```python
from build123d import *

# Parameters (mm, degrees)
ESQUISSE1_R      = 72.5
ESQUISSE1_R_2    = 5
ESQUISSE1_R_3    = 2
EXTRUSION1_DEPTH = 30


with BuildPart() as part:
    # Esquisse1 → Extrusion1 (new body)
    with BuildSketch(Plane.XY):
        Circle(ESQUISSE1_R)
        with Locations((0, -65)):
            Circle(ESQUISSE1_R_2, mode=Mode.SUBTRACT)
        with Locations((65, 0)):
            Circle(ESQUISSE1_R_2, mode=Mode.SUBTRACT)
        with Locations((0, 65)):
            Circle(ESQUISSE1_R_2, mode=Mode.SUBTRACT)
        with Locations((32.5, 56.291651246)):
            Circle(ESQUISSE1_R_3, mode=Mode.SUBTRACT)
        with Locations((-32.5, -56.291651246)):
            Circle(ESQUISSE1_R_3, mode=Mode.SUBTRACT)
        with Locations((-65, 0)):
            Circle(ESQUISSE1_R_2, mode=Mode.SUBTRACT)
    extrude(amount=-EXTRUSION1_DEPTH)

    # Esquisse2 → Enlèvement de matière-Révolution1 (revolve, cut)
    with BuildSketch(Plane(origin=(0, 0, 0), x_dir=(0, 0, -1), z_dir=(1, 0, 0)), mode=Mode.PRIVATE) as enl_vement_de_mati_re_r_volution1_sk:
        Polygon((14, 15), (15, 15.577350269), (15, 17.5), (21, 17.5), (22, 18.077350269), (22, 18.5), (30, 18.5), (30, -2.5), (0, -2.5), (0, 18.077350269), (1, 17.5), (3, 17.5), (3, 15), (4, 15), (4, 11.5), (6, 11.5), (6, 15), align=None)
    revolve(enl_vement_de_mati_re_r_volution1_sk.sketch.rotate(Axis((0, -2.5, 0), (0, 0, -1)), 180), axis=Axis((0, -2.5, 0), (0, 0, -1)), mode=Mode.SUBTRACT)  # turned: the seam where the file's is

    # Esquisse3 → Enlèvement de matière-Révolution2 (revolve, cut)
    with BuildSketch(Plane(origin=(0, 0, 0), x_dir=(0, 0, -1), z_dir=(1, 0, 0))):
        Polygon((10, -41.5), (10, -45.5), (20, -45.5), (20, -51.5), (10, -51.5), (10, -55.5), (20, -55.5), (20, -82.5), (0, -82.5), (0, -30.5), (10, -30.5), (10, -35.5), (20, -35.5), (20, -41.5), align=None)
    revolve(axis=Axis((0, -2.5, 12.602017423), (0, 0, -1)), mode=Mode.SUBTRACT)


solid = part.part
```
Can you work these out from the model? Positions are in its coordinate system, mm. A direction names the side the tool comes from. Round coordinates to 2 decimals unless told otherwise and drop trailing zeros. Loops run counter-clockwise (first coordinate to the right, second up) from the corner with the lowest first, then second, coordinate; pieces in that order, holes last. Notation, with made-up numbers: (29, 57.5) -> (88, 57.5) arc R9 ccw to (88, 72.5) -> close; hole circle Ø6 at (81, -13). An arc over 180 degrees is marked (long way). One line per item, written item: value. Start each with the question number.
1. If I drill on probe 1 along X at (y, z) = (-2.5, -16.25); probe 2 along Y at (x, z) = (40, -16.5); probe 3 along Y at (x, z) = (15, -15.5), over which ranges is the centre line in solid material (lowest first)?
2. If we section it at D-D, the plane y = 0: Give the number of separate pieces and of enclosed holes in the cut face, then the cut area to 3 significant figures.
3. For pin 1 (8 mm diameter, centred on x = 0, y = -65, fed in from -Z); pin 2 (4 mm diameter, centred on x = -5.5, y = 52.5, fed in from +Z); pin 3 (5 mm diameter, centred on x = 3, z = -7, fed in from +Y); pin 4 (4 mm diameter, centred on x = 13.5, y = -3.5, fed in from -Z), each with a flat end and sliding along its axis, tell me the tip position at first contact or that it passes through.
4. If we section it at A-A, the plane z = -18: Write out the boundary of the cut face in (x, y).
5. If we section it at B-B, the plane x = -65: Write out the boundary of the cut face in (y, z).
6. For faces 4 (the flat face through (-8.8, -34.5, -20)), 5 (the cylindrical face through (69.15, 21.78, -24.93)), 6 (the cylindrical face through (-6.007, -21.576, -18.042)), which set-ups out of +Z, -Z, +X, -X, +Y, -Y let a thin tool reach every point of the face, with its end or its side?
7. If we mould it in two halves opening along Y, with no side actions, what happens to faces 1 (the cylindrical face through (-44.69, -30.99, -15.07)), 2 (the flat face through (-15, 12, 0)), 3 (the cylindrical face through (-70, 0, -25))? For each: pulls with the +Y half, pulls with the -Y half, needs draft (parallel to the pull), parting line crosses it, or undercut.
Calculated:
1. probe 1: x = -53 to -49, -43 to -39, -33 to -20, 20 to 33, 39 to 43, 49 to 53
1. probe 2: y = -37.27 to -30.8, -18.28 to 13.28, 25.8 to 32.27
1. probe 3: y = -53.33 to -49.15, -42.8 to -38.5, -31.89 to -15.73, 10.73 to 26.89, 33.5 to 37.8, 44.15 to 48.33
2. separate pieces: 4
2. enclosed holes: 0
2. area: 1,490 mm²
3. pin 1: passes through
3. pin 2: stops at z = -20
3. pin 3: stops at y = 25.5
3. pin 4: stops at z = -6
4. outline: circle Ø106 at (0, -2.5); circle Ø86 at (0, -2.5); circle Ø66 at (0, -2.5); hole circle Ø98 at (0, -2.5); hole circle Ø78 at (0, -2.5); hole circle Ø40 at (0, -2.5)
5. outline: (-32.11, -30) -> (-5, -30) -> (-5, -20) -> (-32.11, -20) -> close; (5, -30) -> (32.11, -30) -> (32.11, -20) -> (5, -20) -> close
6. face 4: +Z
6. face 5: +Z, -Z
6. face 6: -Z
7. face 1: parting line crosses it
7. face 2: needs draft
7. face 3: undercut
